Here's how the part is built. I have some questions about the finished solid (model axes, mm). A direction names the side the tool comes from. Round coordinates to 2 decimals unless told otherwise and drop trailing zeros. Order: outer loops, then holes, each group sorted by start corner. A loop starts at its lowest first (then second) coordinate and runs counter-clockwise, first axis right, second up. Notation, with made-up numbers: M 7,-25 L 20,-25 A35 ccw 20,8 Z; hole C -33.75,89 d6. An arc over 180 degrees is marked long. Write item = value, one per line. Start each with the question number.
Item 1: For faces 1 (the face through (35, 599, 980)), 2 (the face through (30.926, 490.934, 592.637)), which set-ups out of +Z, -Z, +X, -X, +Y, -Y let a thin tool reach every point of the face, with its end or its side?
Item 2: I want a section at C-C, the plane x = -18.5. List the corners of the cut face in (y, z) for me.
Item 3: I'm going to push flat-ended pins straight in: P1, Ø8, axis at y = 310, z = 210, coming from the +X side; P2, Ø1, axis at x = -5.5, z = 859.5, coming from the +Y side. Where does each tip first touch, or does it pass through?
Item 4: Please list where these lines run through material, in increasing order: L1, parallel to X at y = 891, z = 835; L2, parallel to X at y = 899.5, z = 642.5; L3, parallel to Y at x = -40, z = 669.
Item 5: I want a section at B-B, the plane y = 230.5. List the corners of the cut face in (x, z) for me.
Item 6: I want a section at D-D, the plane z = 736. List the corners of the cut face in (x, y) for me.
Item 7: I want a section at A-A, the plane z = 406. List the corners of the cut face in (x, y) for me, plus the area to 3 significant figures.
Autodesk Inventor part; units mm, degrees
ref_plane "YZ Plane" through (0, 0, 0) normal (1, 0, 0) x (0, 1, 0)
ref_plane "XZ Plane" through (0, 0, 0) normal (0, 1, 0) x (-1, 0, 0)
ref_plane "XY Plane" through (0, 0, 0) normal (0, 0, 1) x (1, 0, 0)
sketch "Sketch1" plane through (0, 0, 0) normal (0, 0, 1) x (1, 0, 0)
  line L0 (8972.064376, -2416.982713) -> (8972.064376, -2466.982713) construction
  line L1 (0, 47) -> (0, 0) construction
  arc A0 (0.159434, 1.869277) -> (0, 1880) centre (-11009.945504, 940) ccw
  arc A1 (0, 0) -> (0.159434, 1.869277) centre (-11009.945504, 940) ccw construction
  arc A2 (-1.349222, -1.302929) -> (0.159434, 1.869277) centre (-4.822514, 2.29377) ccw
  line L2 (-1.349222, -1.302929) -> (0, 0) construction
  line L3 (-46.757087, -45.152794) -> (-1.349222, -1.302929)
  line L4 (-41.190716, -50.91694) -> (-46.757087, -45.152794) construction
  line L5 (0, 0) -> (0, 1880) construction
  line L6 (0, 0) -> (1.875639, 0) construction
  dimension "d154" = 5
  dimension "d155" = 65
  dimension "d156" = 11050
  dimension "d157" = 136
  dimension "d158" = 1880
contour flange "Contour Flange2" sketch "Sketch1" thickness 3 bend radius 3 width 980 along (0, 0, 1) mid plane no both sides no wall seen from (-24.053155, -23.227861, 0) lies toward (0.6946584, -0.7193398, 0) curves L3 A2 A0
bend "Bend2"
corner "Corner2"
sketch "Sketch5" plane through (0, 0, 0) normal (1, 0, 0) x (0, 1, 0)
  line L0 (1.614581, 980) -> (1.614581, 0)
  line L1 (1.614581, 0) -> (1880.255204, 0)
  line L2 (1880.255204, 0) -> (1880.255204, 980)
  line L3 (1.614581, 980) -> (1880.255204, 980)
  line L4 (1.614581, 980) -> (1.614581, 0)
  line L5 (-3.460948, 980) -> (1.614581, 980)
  line L6 (-3.460948, 980) -> (-3.460948, 0)
  line L7 (-3.460948, 0) -> (1.614581, 0)
  line L8 (-3.460948, 980) -> (-3.460948, 0)
  line L9 (-47.310813, 980) -> (-3.460948, 980)
  line L10 (-47.310813, 0) -> (-47.310813, 980)
  line L11 (-47.310813, 0) -> (-3.460948, 0)
  line L12 (1238.605204, 0) -> (416.287565, 980)
  line L13 (419.406335, 980) -> (-47.310813, 588.377813)
  line L14 (419.406335, 0) -> (-47.310813, 391.622187)
  line L15 (416.287565, 0) -> (1238.605204, 980)
  point P0 (0, 0)
  point P1 (-3.460948, 0)
  point P2 (1.614581, 0)
  dimension "d161" = 40
  dimension "d162" = 40
  dimension "d163" = 641.65
  dimension "d164" = 641.65
  dimension "d166" = 300
  dimension "d167" = 300
extrude "Extrusion3" cut sketch "Sketch5" along normal through all both and the other way through all contours L14 L15 L1 L0 | L0 L7 L6 L14 | L15 L12 L1 L14 | L14 L1 L15 | L6 L11 L10 L14 | L15 L3 L2 L1 L12
sketch "Sketch8" plane through (-1.349222, -1.302929, 980) normal (-0.6946584, 0.7193398, 0) x (0.7193398, 0.6946584, 0)
  line L0 (-39.124361, 25.740843) -> (-51.124361, 25.740843) construction
  line L1 (-51.124361, 25.740843) -> (-51.124361, 162.747026) construction
  line L2 (-51.124361, 162.747026) -> (-39.124361, 162.747026) construction
  line L3 (-39.124361, 162.747026) -> (-39.124361, 25.740843) construction
  line L4 (-63.124361, 0) -> (-63.124361, 590.188606)
  point P0 (1.875639, 980)
  dimension "d168" = 12
  dimension "d169" = 12
mark "Mark5"
equation "\"d36\" = Thickness"
equation "\"d37\" = BendReliefWidth"
equation "\"d38\" = BendReliefDepth"
equation "\"d39\" = MinimumRemnant"
equation "\"d40\" = TransitionRadius"
equation "\"d42\" = BendRadius"
equation "\"d44\" = CornerReliefSize"
equation "\"d45\" = GapSize"
equation "\"d46\" = JacobiRadiusSize"
equation "\"BendRadius\" = Thickness"
equation "\"BendReliefWidth\" = Thickness"
equation "\"BendReliefDepth\" = 0.5 * Thickness"
equation "\"CornerReliefSize\" = 4 * Thickness"
equation "\"MinimumRemnant\" = 2 * Thickness"
equation "\"TransitionRadius\" = BendRadius"
equation "\"JacobiRadiusSize\" = BendRadius"
equation "\"GapSize\" = Thickness"
properties part number "MSC 304 sheet right board face" material "AISI304"
Filled in:
q1.face_1 = +Z, +X, -X, +Y, -Y
q1.face_2 = +Z, -Z, -X
q2.outline = M -22.04,370.41 L -17.87,366.91 L -17.87,980 L -22.04,980 Z
q3.P1 = 25.31
q3.P2 = -4.83
q4.L1 = 39.95 to 42.95
q4.L2 = 39.98 to 42.98
q4.L3 = -42.8 to -38.63
q5.outline = M 17.25,158.51 L 20.26,158.51 L 20.26,980 L 17.25,980 Z
q6.outline = M -46.76,-45.15 L -44.67,-47.31 L 0.73,-3.46 A8 ccw 3.15,1.61 A11053 ccw 42.66,1033.86 L 39.66,1033.86 A11050 cw 0.16,1.87 A5 cw -1.35,-1.3 Z
q7.outline = M -46.76,-45.15 L -44.67,-47.31 L 0.73,-3.46 A8 ccw 3.15,1.61 A11053 ccw 41.54,756.96 L 38.54,756.96 A11050 cw 0.16,1.87 A5 cw -1.35,-1.3 Z
q7.area = 2,470 mm^2
